Autodesk Inventor part; units mm, degrees
ref_plane "YZ Plane" through (0, 0, 0) normal (1, 0, 0) x (0, 1, 0)
ref_plane "XZ Plane" through (0, 0, 0) normal (0, 1, 0) x (-1, 0, 0)
ref_plane "XY Plane" through (0, 0, 0) normal (0, 0, 1) x (1, 0, 0)
sketch "Szkic1" plane through (0, 0, 0) normal (0, 0, 1) x (1, 0, 0)
  line L0 (260, 0) -> (-260, 0) construction
  line L1 (260, 6) -> (-260, 6)
  line L2 (-260, -6) -> (260, -6)
  arc A0 (260, -6) -> (260, 6) centre (260, 0) ccw
  arc A1 (-260, 6) -> (-260, -6) centre (-260, 0) ccw
  line L3 (-260, 7.4) -> (260, 7.4)
  arc A2 (260, -7.4) -> (260, 7.4) centre (260, 0) ccw
  line L4 (260, -7.4) -> (-260, -7.4)
  arc A3 (-260, 7.4) -> (-260, -7.4) centre (-260, 0) ccw
  point P0 (0, 0)
  dimension "d0" = 260
  dimension "d1" = 12
  dimension "d2" = 1.4
extrude "Wyciągnięcie proste1" add sketch "Szkic1" along normal blind 6.3
properties part number "COTS_GENERIC_Y_Axis_Timing_Belt"
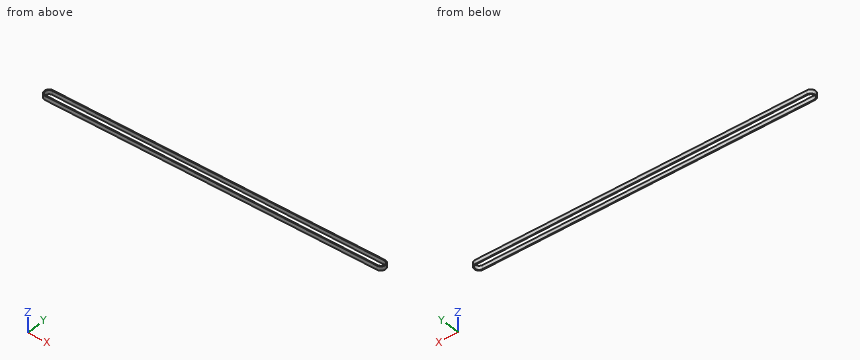
For this review, take the finished solid that the model builds, in its own axes (mm). Give positions to 0.01 mm unless a question says otherwise; leave off trailing zeros. Loops run counter-clockwise (first coordinate to the right, second up) from the corner with the lowest first, then second, coordinate; pieces in that order, holes last.
Item 1: For line 1 along Y through (x, z) = (-21, 5.75); line 2 along X through (y, z) = (-4, 2.5); line 3 along X through (y, z) = (-3.25, 4.75), list the stretches that pass through material, from the lowest coordinate up.
Item 2: Take a section at C-C, the plane z = 1. State the section outline as (x, y) points.
Item 3: Insertion check: pin 1 (1 mm diameter, centred on y = -2.5, z = 4, fed in from +X); pin 2 (6 mm diameter, centred on x = -58, y = -4.5, fed in from +Z). Each pin has a flat end and moves straight along its axis. Give the tip position at first contact, or say it passes through.
Item 4: Take a section at A-A, the plane x = 229. State the section outline as (y, z) points.
Item 5: Take a section at B-B, the plane y = 0. State the section outline as (x, z) points.
Calculated:
1. line 1: y = -7.4 to -6, 6 to 7.4
1. line 2: x = -266.23 to -264.47, 264.47 to 266.23
1. line 3: x = -266.65 to -265.04, 265.04 to 266.65
2. outline: (-260, -7.4) - (260, -7.4) arc R7.4 ccw to (260, 7.4) - (-260, 7.4) arc R7.4 ccw to start; hole (-260, -6) - (260, -6) arc R6 ccw to (260, 6) - (-260, 6) arc R6 ccw to start
3. pin 1: stops at x = 267.12
3. pin 2: stops at z = 6.3
4. outline: (-7.4, 0) - (-6, 0) - (-6, 6.3) - (-7.4, 6.3) - close; (6, 0) - (7.4, 0) - (7.4, 6.3) - (6, 6.3) - close
5. outline: (-267.4, 0) - (-266, 0) - (-266, 6.3) - (-267.4, 6.3) - close; (266, 0) - (267.4, 0) - (267.4, 6.3) - (266, 6.3) - close
